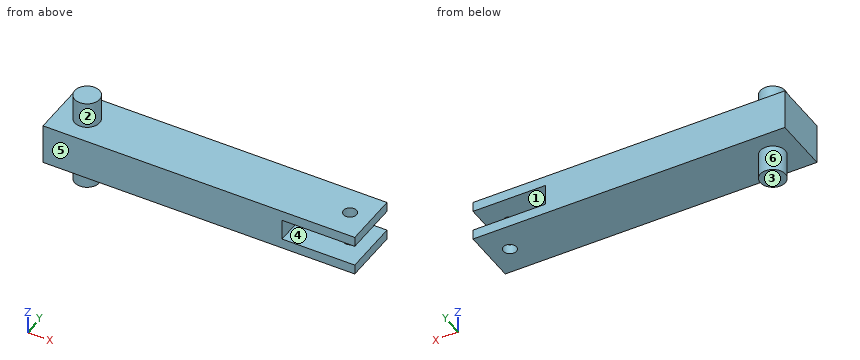
```python
from build123d import *

# Parameters (mm, degrees)
SKETCH1_W           = 600
SKETCH1_H           = 78
BOSS_EXTRUDE1_DEPTH = 108
SKETCH2_R           = 24
BOSS_EXTRUDE2_DEPTH = 50
BOSS_EXTRUDE3_START = 50
SKETCH3_R           = 24
BOSS_EXTRUDE3_DEPTH = 50
SKETCH4_W           = 140
SKETCH4_H           = 40
CUT_EXTRUDE1_DEPTH  = 332.036251791
SKETCH5_R           = 12.5
CUT_EXTRUDE2_DEPTH  = 344.581140344


with BuildPart() as part:
    # Sketch1 → Boss-Extrude1 (new body)
    with BuildSketch(Plane(origin=(0, 0, 0), x_dir=(1, 0, 0), z_dir=(0, 1, 0))):
        Rectangle(SKETCH1_W, SKETCH1_H)
    extrude(amount=BOSS_EXTRUDE1_DEPTH)

    # Sketch2 → Boss-Extrude2 (add)
    with BuildSketch(Plane.XY.offset(39)):
        with Locations(Location((-246, 54, 0), (0, 0, 180))):
            Circle(SKETCH2_R)
    extrude(amount=BOSS_EXTRUDE2_DEPTH)

    # Sketch3 → Boss-Extrude3 (add)
    with BuildSketch(Plane(origin=(0, 0, -39), x_dir=(-1, 0, 0), z_dir=(0, 0, -1)).offset(BOSS_EXTRUDE3_START)):
        with Locations((246, 54)):
            Circle(SKETCH3_R)
    extrude(amount=-BOSS_EXTRUDE3_DEPTH)

    # Sketch4 → Cut-Extrude1 (cut, through all)
    with BuildSketch(Plane(origin=(0, 0, 0), x_dir=(-1, 0, 0), z_dir=(0, -1, 0))):
        with Locations((-230, 0)):
            Rectangle(SKETCH4_W, SKETCH4_H)
    extrude(amount=-CUT_EXTRUDE1_DEPTH, mode=Mode.SUBTRACT)

    # Sketch5 → Cut-Extrude2 (cut, through all)
    with BuildSketch(Plane(origin=(0, 0, -39), x_dir=(-1, 0, 0), z_dir=(0, 0, -1))):
        with Locations((-260, 54)):
            Circle(SKETCH5_R)
    extrude(amount=-CUT_EXTRUDE2_DEPTH, mode=Mode.SUBTRACT)


solid = part.part
```
Model file for the job. Use its own axes, mm. Face numbers are marked on the shaded views. A direction names the side the tool comes from. Give positions to 0.01 mm unless a question says otherwise; leave off trailing zeros. Loops run counter-clockwise (first coordinate to the right, second up) from the corner with the lowest first, then second, coordinate; pieces in that order, holes last. Notation, with made-up numbers: M 64,-11.75 L 71,-11.75 A32 cw 71,24.25 Z; hole C 28,58.25 d2. An arc over 180 degrees is marked long. Use one line per item in the form item = value.
Item 1: Which spindle directions (+Z, -Z, +X, -X, +Y, -Y) get a long thin tool onto all of the face, cutting with end or side? Do the marked faces 4, 5 and 6. Say none if no direction does.
Filled in:
face_4 = +X, +Y, -Y
face_5 = +Z, -Z, +X, -X, -Y
face_6 = -Z
Item 2: Flat gauge pins, fed straight in: pin 1 Ø4 at (x, y) = (112, 37.5) entering from -Z; pin 2 Ø6 at (y, z) = (37, 4) entering from +X. Where does each tip first touch, or does it go through?
Filled in:
pin_1 = -39
pin_2 = 160
Item 3: Slice it at A-A on y = 54. List the corners of the cut face in (x, z), and give its area (4 significant figures).
Filled in:
outline = M -300,-39 L -270,-39 L -270,-89 L -222,-89 L -222,-39 L 247.5,-39 L 247.5,-20 L 160,-20 L 160,20 L 247.5,20 L 247.5,39 L -222,39 L -222,89 L -270,89 L -270,39 L -300,39 Z; M 272.5,-39 L 300,-39 L 300,-20 L 272.5,-20 Z; M 272.5,20 L 300,20 L 300,39 L 272.5,39 Z
area = 45,050 mm^2
Item 4: Two-plate mould, pull along Z, no slides. Class the marked faces 1, 2 and 3: released by +Z, released by -Z, zero draft, split by the parting line, or undercut.
Filled in:
face_1 = undercut
face_2 = zero draft
face_3 = released by -Z
Item 5: Slice it at D-D on x = -246. List the corners of the cut face in (y, z).
Filled in:
outline = M 0,-39 L 30,-39 L 30,-89 L 78,-89 L 78,-39 L 108,-39 L 108,39 L 78,39 L 78,89 L 30,89 L 30,39 L 0,39 Z
Item 6: Slice it at C-C on y = 95. List the corners of the cut face in (x, z).
Filled in:
outline = M -300,-39 L 300,-39 L 300,-20 L 160,-20 L 160,20 L 300,20 L 300,39 L -300,39 Z
Item 7: Drill centre lines: L1, parallel to Y at x = 260, z = 34; L2, parallel to Z at x = 238, y = 35.5; L3, parallel to Z at x = -55, y = 49.5. Where is each one in solid material? Low to high.
Filled in:
L1 = 0 to 41.5, 66.5 to 108
L2 = -39 to -20, 20 to 39
L3 = -39 to 39
Item 8: Slice it at B-B on x = 260. List the corners of the cut face in (y, z), and give its area (3 significant figures).
Filled in:
outline = M 0,-39 L 41.5,-39 L 41.5,-20 L 0,-20 Z; M 0,20 L 41.5,20 L 41.5,39 L 0,39 Z; M 66.5,-39 L 108,-39 L 108,-20 L 66.5,-20 Z; M 66.5,20 L 108,20 L 108,39 L 66.5,39 Z
area = 3,150 mm^2
